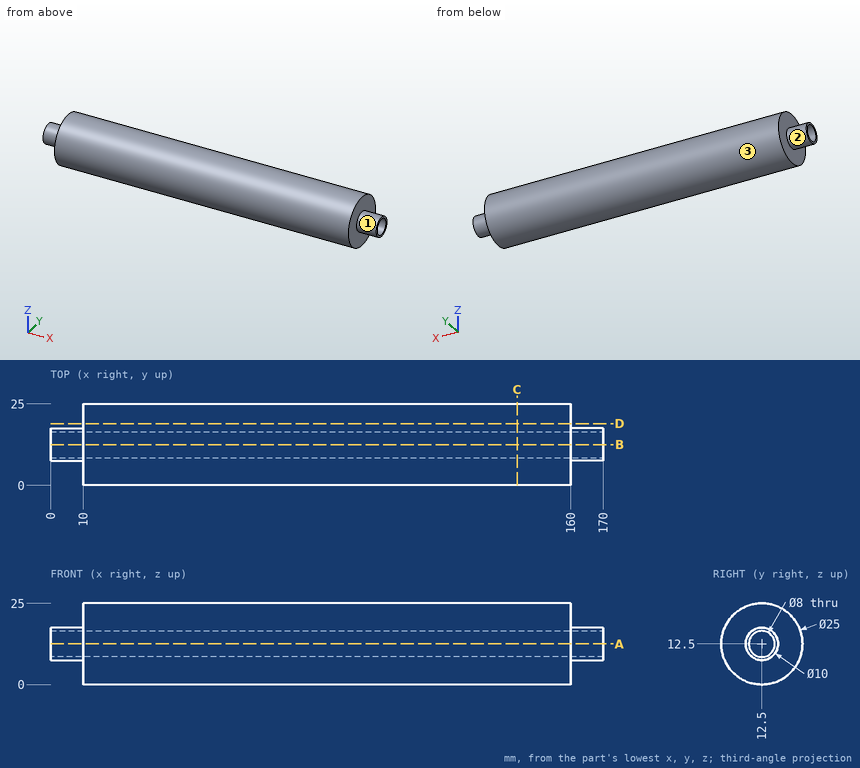
Part print with two shaded views. Sizes in mm from the minimum x, y, z corner. A direction names the side the tool comes from. Round coordinates to 2 decimals unless told otherwise and drop trailing zeros. Loops run counter-clockwise (first coordinate to the right, second up) from the corner with the lowest first, then second, coordinate; pieces in that order, holes last.
1. Flat gauge pins, fed straight in: pin 1 (1.5 mm diameter, centred on y = 11.5, z = 20, fed in from -X); pin 2 (4 mm diameter, centred on x = 137, z = 13.5, fed in from +Y); pin 3 (6 mm diameter, centred on x = 65, z = 16, fed in from -Y); pin 4 (4 mm diameter, centred on x = 137, z = 7.5, fed in from -Y). Where does each tip first touch, or does it go through?
Solutions:
pin 1: stops at x = 10
pin 2: stops at y = 25
pin 3: stops at y = 0.01
pin 4: stops at y = 0.37
2. Slice it at C-C (x = 143.5). Give the cut face in (y, z), and give its area (3 significant figures).
Solutions:
outline: circle Ø25 at (12.5, 12.5); hole circle Ø8 at (12.5, 12.5)
area: 441 mm2
3. Slice it at D-D (y = 19). Give the cut face in (x, z).
Solutions:
outline: (10, 1.82) - (160, 1.82) - (160, 23.18) - (10, 23.18) - close
4. Drill centre lines: line 1 along Y through (x, z) = (44.5, 12.5); line 2 along X through (y, z) = (12, 2.75); line 3 along Z through (x, y) = (126.5, 9). Where is each one in solid material? Low to high.
Solutions:
line 1: y = 0 to 8.5, 16.5 to 25
line 2: x = 10 to 160
line 3: z = 0.5 to 10.56, 14.44 to 24.5
5. Slice it at A-A (z = 12.5). Give the cut face in (x, y), and give its area (3 significant figures).
Solutions:
outline: (0, 7.5) - (10, 7.5) - (10, 0) - (160, 0) - (160, 7.5) - (170, 7.5) - (170, 8.5) - (0, 8.5) - close; (0, 16.5) - (170, 16.5) - (170, 17.5) - (160, 17.5) - (160, 25) - (10, 25) - (10, 17.5) - (0, 17.5) - close
area: 2,590 mm2
6. 3-axis set-ups, long thin cutter, end or side, ignore diameter. For the marked faces 1, 2 and 3: which of +Z, -Z, +X, -X, +Y, -Y reach the whole face in a straight line?
Solutions:
face 1: +X
face 2: -X
face 3: +X, -X
